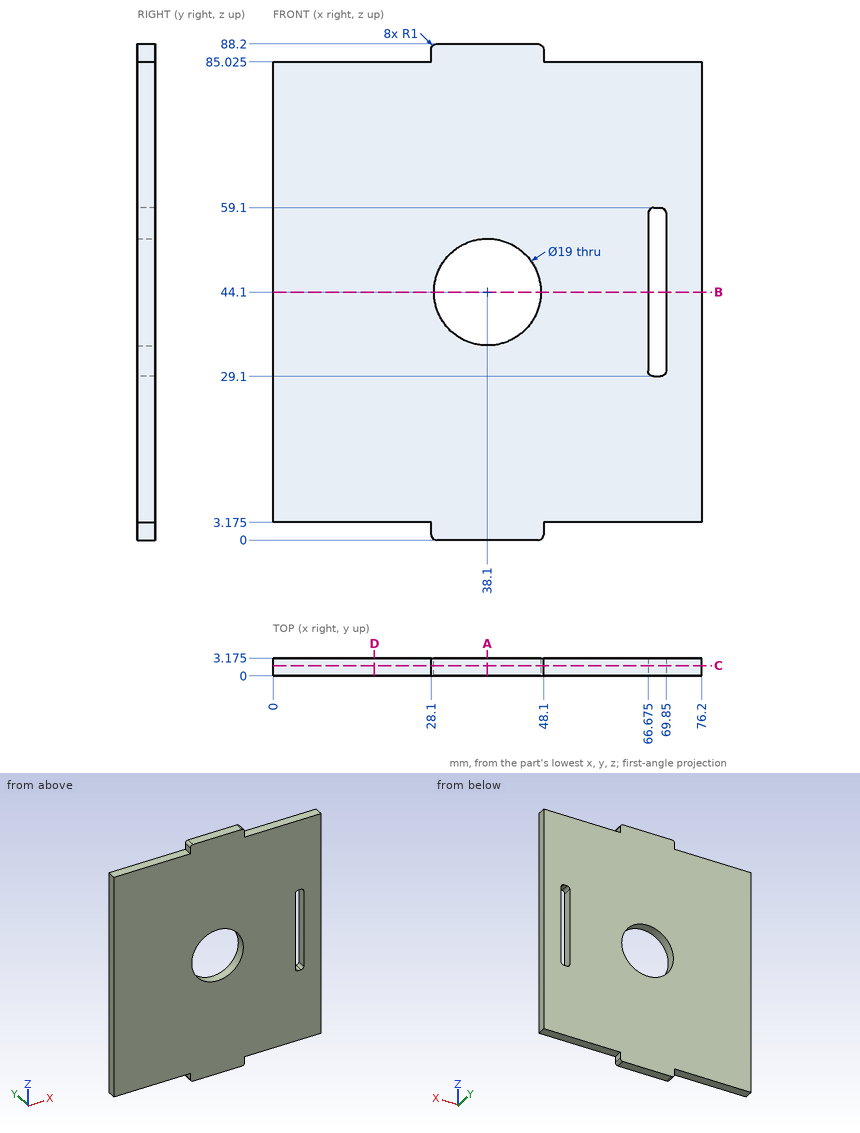
The drawing under review shows one solid part. Ordinate dimensions are in mm from its lowest x, y, z. Give positions to 0.01 mm unless a question says otherwise; leave off trailing zeros. Write each loop counter-clockwise with the first axis right and the second up, starting at its lowest first coordinate (ties: lowest second). Pieces come first, ordered by that corner, then holes. Notation, with made-up numbers: M -11,-27 L 30,-27 A20 cw 30,-15 Z; hole C 44.5,70.25 d7. An arc over 180 degrees is marked long. Write each question's results on one line, items separated by ' | '. Start each with the question number.
1. We need section B-B (z = 44.1). Write out the cut boundary in (x, y) (3 decimals).
2. For probe 1 along X at (y, z) = (2.5, 44.1) (3 decimals); probe 2 along Z at (x, y) = (38.1, 1.7); probe 3 along X at (y, z) = (2.5, 31) (3 decimals), list the stretches that pass through material, from the lowest coordinate up. Write a range as [from, to].
3. We need section D-D (x = 18). Write out the cut boundary in (y, z) (3 decimals), and give its area (3 significant figures).
4. Insertion check: pin 1 Ø0.7 at (y, z) = (2, 2) entering from -X; pin 2 Ø1 at (x, y) = (8.5, 1.5) entering from -Z (3 decimals); pin 3 Ø2 at (x, z) = (28, 34) entering from -Y; pin 4 Ø0.9 at (x, y) = (68.5, 1) entering from +Z (3 decimals). Each pin has a flat end and moves straight along its axis. Give the tip position at first contact, or say it passes through.
5. We need section C-C (y = 1.85). Write out the cut boundary in (x, z) (3 decimals), and give its area (3 significant figures).
6. We need section A-A (x = 38.1). Write out the cut boundary in (y, z) (3 decimals).
Results found:
1) outline: M 0,0 L 28.6,0 L 28.6,3.175 L 0,3.175 Z; M 47.6,0 L 66.675,0 L 66.675,3.175 L 47.6,3.175 Z; M 69.85,0 L 76.2,0 L 76.2,3.175 L 69.85,3.175 Z
2) probe 1: x = [0, 28.6], [47.6, 66.675], [69.85, 76.2] | probe 2: z = [0, 34.6], [53.6, 88.2] | probe 3: x = [0, 66.675], [69.85, 76.2]
3) outline: M 0,3.175 L 3.175,3.175 L 3.175,85.025 L 0,85.025 Z | area: 260 mm^2
4) pin 1: stops at x = 28.1 | pin 2: stops at z = 3.175 | pin 3: stops at y = 0 | pin 4: stops at z = 85.025
5) outline: M 0,3.175 L 28.1,3.175 L 28.1,1 A1 ccw 29.1,0 L 47.1,0 A1 ccw 48.1,1 L 48.1,3.175 L 76.2,3.175 L 76.2,85.025 L 48.1,85.025 L 48.1,87.2 A1 ccw 47.1,88.2 L 29.1,88.2 A1 ccw 28.1,87.2 L 28.1,85.025 L 0,85.025 Z; hole C 38.1,44.1 d19; hole M 66.675,30.1 A1 ccw 67.675,29.1 L 68.85,29.1 A1 ccw 69.85,30.1 L 69.85,58.1 A1 ccw 68.85,59.1 L 67.675,59.1 A1 ccw 66.675,58.1 Z | area: 5,990 mm^2
6) outline: M 0,0 L 3.175,0 L 3.175,34.6 L 0,34.6 Z; M 0,53.6 L 3.175,53.6 L 3.175,88.2 L 0,88.2 Z
